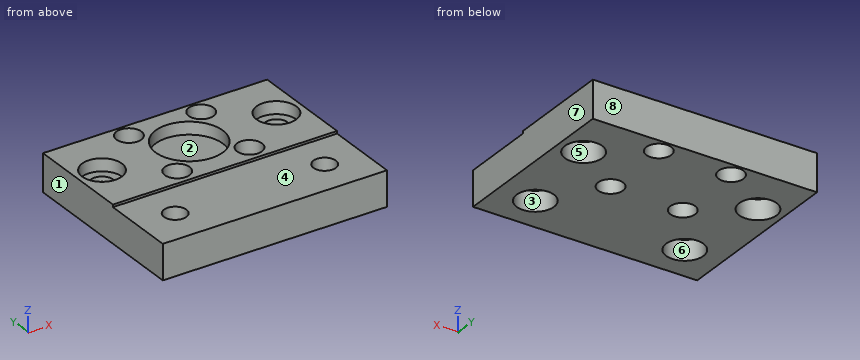
```python
from build123d import *

# Parameters (mm, degrees)
SKETCH1_W                      = 90
SKETCH1_H                      = 72
BOSS_EXTRUDE1_DEPTH            = 15
SKETCH2_W                      = 90
SKETCH2_H                      = 30
CUT_EXTRUDE1_DEPTH             = 1
SKETCH3_R                      = 5
CUT_EXTRUDE2_DEPTH             = 60.548299724
SKETCH4_R                      = 13.5
SKETCH4_R_2                    = 8
CUT_EXTRUDE3_DEPTH             = 5
CBORE_FOR_M8_SHCS1_D           = 9
CBORE_FOR_M8_SHCS1_DEPTH       = 15
CBORE_FOR_M8_SHCS1_CBORE_D     = 15
CBORE_FOR_M8_SHCS1_CBORE_DEPTH = 8
CBORE_FOR_M8_SHCS1_TIP         = 2.703872786


with BuildPart() as part:
    # Sketch1 → Boss-Extrude1 (new body)
    with BuildSketch(Plane.XY):
        Rectangle(SKETCH1_W, SKETCH1_H)
    extrude(amount=BOSS_EXTRUDE1_DEPTH)

    # Sketch2 → Cut-Extrude1 (cut)
    with BuildSketch(Plane.XY.offset(15)):
        with Locations((0, -21)):
            Rectangle(SKETCH2_W, SKETCH2_H)
    extrude(amount=-CUT_EXTRUDE1_DEPTH, mode=Mode.SUBTRACT)

    # Sketch3 → Cut-Extrude2 (cut, through all)
    with BuildSketch(Plane.XY.offset(15)):
        with Locations((-14.5, 30)):
            Circle(SKETCH3_R)
        with Locations((14.5, 30)):
            Circle(SKETCH3_R)
        with Locations((14.5, 1)):
            Circle(SKETCH3_R)
        with Locations((-14.5, 1)):
            Circle(SKETCH3_R)
    extrude(amount=-CUT_EXTRUDE2_DEPTH, mode=Mode.SUBTRACT)

    # Sketch4 → Cut-Extrude3 (cut)
    with BuildSketch(Plane.XY.offset(15)):
        with Locations((0, 15.5)):
            Circle(SKETCH4_R)
        with Locations((-35, 15.5)):
            Circle(SKETCH4_R_2)
        with Locations(Location((35, 15.5, 0), (0, 0, 180))):
            Circle(SKETCH4_R_2)
    extrude(amount=-CUT_EXTRUDE3_DEPTH, mode=Mode.SUBTRACT)

    # CBORE for M8 SHCS1
    with Locations(Plane(origin=(0, 0, 0), x_dir=(-1, 0, 0), z_dir=(0, 0, -1))):
        with Locations((30, -21), (-30, -21), (-35, 15.5), (35, 15.5)):
            CounterBoreHole(CBORE_FOR_M8_SHCS1_D / 2, CBORE_FOR_M8_SHCS1_CBORE_D / 2, CBORE_FOR_M8_SHCS1_CBORE_DEPTH, depth=CBORE_FOR_M8_SHCS1_DEPTH)
            with Locations((0, 0, -(CBORE_FOR_M8_SHCS1_DEPTH + CBORE_FOR_M8_SHCS1_TIP / 2))):  # 118° drill point
                Cone(0, CBORE_FOR_M8_SHCS1_D / 2, CBORE_FOR_M8_SHCS1_TIP, mode=Mode.SUBTRACT)


solid = part.part
```
Source: CAD feature listing. Evaluate the final solid. Frame: model axes, mm. Face numbers are marked on the shaded views. A direction names the side the tool comes from. Round coordinates to 2 decimals unless told otherwise and drop trailing zeros. Loops run counter-clockwise (first coordinate to the right, second up) from the corner with the lowest first, then second, coordinate; pieces in that order, holes last. Notation, with made-up numbers: M 38,-17.5 L 63,-17.5 A26 ccw 63,11.5 Z; hole C -4,-25.5 d10. An arc over 180 degrees is marked long. Use a Markdown table: item, result. Add a question column.
1. Cut plane B-B, the plane y = 30. Output: boundary loops of the cut face in (x, z), and give its area (3 significant figures).
2. Cut plane A-A, the plane x = -18.5. Output: boundary loops of the cut face in (y, z), and give its area (3 significant figures).
3. Pull-direction query (Y, two-part tool) for the marked faces 5, 6, 7 and 8; classes: +Y half, -Y half, draft (parallel to the pull), parting line (faces both ways), or undercut.
4. Ray query, line 1 along X through (y, z) = (16, 11.5); line 2 along Y through (x, z) = (-14, 3.5); line 3 along Y through (x, z) = (-30, 3.75). Return the intervals inside material, ascending. Write a range as [from, to].
5. Contact query for flat-ended pins moving along their axis: pin 1 (12 mm diameter, centred on x = -1, y = 22, fed in from +Z); pin 2 (17.5 mm diameter, centred on x = 38, y = 12, fed in from +Z); pin 3 (24 mm diameter, centred on x = 30, y = -21, fed in from +Z); pin 4 (7.5 mm diameter, centred on x = -29.5, y = -23.5, fed in from -Z). Output: stop coordinate, or through.
6. Cut plane D-D, the plane x = 24. Output: boundary loops of the cut face in (y, z), and give its area (3 significant figures).
7. Cut plane C-C, the plane z = 6.25. State how many separate pieces and enclosed holes the cut face has, and give its area (3 significant figures).
8. Set-up query: the marked faces 1, 2, 3 and 4. Return all of +Z, -Z, +X, -X, +Y, -Y with unobstructed straight access to the full face (end or side cutting, diameter ignored); none if empty.
Solution:
| question | item | result |
|---|---|---|
| 1 | outline | M -45,0 L -19.5,0 L -19.5,15 L -45,15 Z; M -9.5,0 L 9.5,0 L 9.5,15 L -9.5,15 Z; M 19.5,0 L 45,0 L 45,15 L 19.5,15 Z |
| 1 | area | 1,050 mm2 |
| 2 | outline | M -36,0 L -2,0 L -2,15 L -6,15 L -6,14 L -36,14 Z; M 4,0 L 27,0 L 27,15 L 4,15 Z; M 33,0 L 36,0 L 36,15 L 33,15 Z |
| 2 | area | 870 mm2 |
| 3 | face 5 | undercut |
| 3 | face 6 | undercut |
| 3 | face 7 | draft |
| 3 | face 8 | +Y half |
| 4 | line 1 | x = [-45, -42.98], [-27.02, -13.49], [13.49, 27.02], [42.98, 45] |
| 4 | line 2 | y = [-36, -3.97], [5.97, 25.03], [34.97, 36] |
| 4 | line 3 | y = [-36, -28.5], [-13.5, 9.91], [21.09, 36] |
| 5 | pin 1 | stops at z = 10 |
| 5 | pin 2 | stops at z = 15 |
| 5 | pin 3 | stops at z = 14 |
| 5 | pin 4 | stops at z = 8 |
| 6 | outline | M -36,0 L -25.5,0 L -25.5,8 L -16.5,8 L -16.5,0 L 36,0 L 36,15 L -6,15 L -6,14 L -36,14 Z |
| 6 | area | 978 mm2 |
| 7 | separate pieces | 1 |
| 7 | enclosed holes | 8 |
| 7 | area | 5,460 mm2 |
| 8 | face 1 | +Z, -Z, -X, +Y, -Y |
| 8 | face 2 | +Z |
| 8 | face 3 | -Z |
| 8 | face 4 | +Z, +X, -X, -Y |
